Autodesk Inventor part; units mm, degrees
ref_plane "Plano de trabajo1" through (86.86, 8.06, 0.025) normal (0, 0, -1) x (-0.9876, 0.157, 0)
ref_plane "YZ Plane" through (0, 0, 0) normal (1, 0, 0) x (0, 1, 0)
ref_plane "XZ Plane" through (0, 0, 0) normal (0, 1, 0) x (-1, 0, 0)
ref_plane "Plano de trabajo1" through (86.86, 8.06, 0.025) normal (0, 0, -1) x (-0.9876, 0.157, 0)
sketch "Boceto1" plane through (86.86, 8.06, 0.025) normal (0, 0, -1) x (-0.9876, 0.157, 0)
  line L0 (0.3099, -7.9427) -> (0.3097, -7.9404)
  circle A0 centre (-0.3141, -1.974) radius 1.9997
  arc A1 (2.1306, 3.5042) -> (0.3097, -7.9404) centre (-0.3141, -1.974) ccw
  arc A2 (76.2508, -20.0134) -> (78.0703, -8.566) centre (78.6942, -14.5335) ccw
  circle A3 centre (78.6942, -14.5335) radius 2
  line L1 (10.4901, -0.1486) -> (9.9896, 0)
  line L2 (69.5109, -9.4609) -> (68.989, -9.4469)
  line L3 (67.8902, -16.3602) -> (68.3907, -16.5087)
  line L4 (9.3912, -7.0618) -> (8.8693, -7.0478)
  line L5 (9.9896, 0) -> (2.1306, 3.5042)
  line L6 (8.8693, -7.0478) -> (0.3097, -7.9404)
  line L7 (9.3912, -7.0618) -> (67.8902, -16.3602)
  line L8 (68.3907, -16.5087) -> (76.2508, -20.0134)
  line L9 (78.0703, -8.566) -> (69.5109, -9.4609)
  line L10 (68.989, -9.4469) -> (10.4901, -0.1486)
  point P0 (84.5179, -21.5953)
  point P1 (2.1295, 3.5047)
  point P2 (78.0703, -8.566)
  point P3 (1.5536, -1.2595)
  point P4 (76.719, -14.2196)
extrude "Extrusión1" add sketch "Boceto1" along normal blind 5
sketch "Boceto2" plane through (86.86, 8.06, 0.025) normal (0, 0, 1) x (0.9876, -0.157, 0)
  point P0 (-84.5179, -21.5953)
properties part number "STEP translator 7.5 1"
Geometry check sheet. Reference: the model listing, model coordinates, mm. A direction names the side the tool comes from. Round coordinates to 2 decimals unless told otherwise and drop trailing zeros. Order: outer loops, then holes, each group sorted by start corner. A loop starts at its lowest first (then second) coordinate and runs counter-clockwise, first axis right, second up. Notation, with made-up numbers: (65.25, 41.5) -> (81.25, 41.5) arc R13 cw to (81.25, 51.5) -> close; hole circle Ø9 at (-30.75, 3.5). An arc over 180 degrees is marked (long way). Use one line per item in the form item = value.
1. Go/stop test with a flat-tipped pin: pin 1 (1 mm diameter, centred on x = 24, z = -1, fed in from +Y). Record where the tip stops, or that it passes through.
Working result:
pin_1 = 9.56
2. Cross-section at A-A, the plane x = 7.5. Enter the section's corners in (y, z) (1 decimal).
Working result:
outline = (0.1, -5) -> (4.2, -5) -> (4.2, 0) -> (0.1, 0) -> close; (8, -5) -> (12, -5) -> (12, 0) -> (8, 0) -> close
3. Scan lines: line 1 along X through (y, z) = (5, -2.05); line 2 along X through (y, z) = (7.75, -4.45); line 3 along Y through (x, z) = (29.5, -4.5). Record each from-to range of solid material in increasing order. Write a range as from..to.
Working result:
line_1 = 0.95..5.17, 8.55..85.17, 88.56..92.76
line_2 = 1.1..5.79, 7.93..85.79, 87.93..92.62
line_3 = 2.56..9.56
4. Set-up check for faces 1 (the face through (12.627, 1.395, -2.44)), 2 (the face through (81.092, 10.726, -2.44)), 3 (the face through (84.88, 5.77, -2.44)): record each of +Z, -Z, +X, -X, +Y, -Y from which the full face is reachable in a straight line by a thin tool's end or side.
Working result:
face_1 = +Z, -Z, -Y
face_2 = +Z, -Z, +Y
face_3 = +Z, -Z
5. Mould release check, pull along X, two halves, no side actions. Record for faces 4 (the face through (4.88, 5.77, -2.44)), 5 (the face through (47, 6, -4.975)): pulls with the +X half, pulls with the -X half, needs draft (parallel to the pull), parting line crosses it, or undercut.
Working result:
face_4 = undercut
face_5 = needs draft
6. Cross-section at C-C, the plane x = 19. Enter the section's corners in (y, z) (3 decimals).
Working result:
outline = (2.561, -4.975) -> (9.561, -4.975) -> (9.561, 0.025) -> (2.561, 0.025) -> close
7. Cross-section at D-D, the plane x = 84. Enter the section's corners in (y, z) (3 decimals), plus the area to 3 significant figures.
Working result:
outline = (0.617, -4.975) -> (11.505, -4.975) -> (11.505, 0.025) -> (0.617, 0.025) -> close
area = 54.4 mm^2
